The model under review builds one solid part; all positions refer to its coordinate system, in mm. A direction names the side the tool comes from. Round coordinates to 2 decimals unless told otherwise and drop trailing zeros. Write each loop counter-clockwise with the first axis right and the second up, starting at its lowest first coordinate (ties: lowest second). Pieces come first, ordered by that corner, then holes. Notation, with made-up numbers: (85.25, 50) -> (128.25, 50) arc R21 ccw to (128.25, 67) -> close; hole circle Ø8 at (55, 41.25). An arc over 180 degrees is marked (long way). Return JSON: item names as keys, results as strings. Group by question number.
1. Take a section at D-D, the plane x = 9. Write out the cut boundary in (y, z).
2. Take a section at A-A, the plane y = -4. Write out the cut boundary in (x, z).
3. Tool access review of faces 3 (the cylindrical face through (0.07, -3.53, 25.5)), 4 (the flat face through (35, 28.6, -20)): name each direction out of +Z, -Z, +X, -X, +Y, -Y from which nothing blocks a thin tool from reaching the whole face with its end or side.
4. For line 1 along Z through (x, y) = (4, -8); line 2 along Y through (x, z) = (-19, -38.5); line 3 along Y through (x, z) = (-32.5, 27), list the stretches that pass through material, from the lowest coordinate up. Write a range as from..to.
5. Take a section at C-C, the plane z = 41. Write out the cut boundary in (x, y), then the cut area to 3 significant figures.
6. Mouldability with a two-part tool opening along Z and no side actions: class faces 1 (the flat face through (-38.1, 22.1, 24.2)), 2 (the cylindrical face through (-4.88, -10.07, -1.08)) as pulls with the +Z half, pulls with the -Z half, needs draft (parallel to the pull), parting line crosses it, or undercut.
7. Clearance check with flat-ended pins moving along their axes: P1, Ø3.5, axis at x = 41.5, z = -0.5, coming from the +Y side; P2, Ø0.9, axis at x = -0.5, z = 27, coming from the +Y side; P3, Ø0.9, axis at x = -34, z = -20.5, coming from the +Y side. State where each tip first meets the part, or that it passes through.
8. Take a section at B-B, the plane y = -11. Write out the cut boundary in (x, z) (1 decimal), then the cut area to 3 significant figures.
from build123d import *

# Parameters (mm, degrees)
SHPERE_HULL_ANGLE    = 180
SKETCH3_W            = 50
SKETCH3_H            = 70
BATTERY_CAVITY_DEPTH = 18.3
SKETCH7_R            = 1.5
CUT_EXTRUDE4_DEPTH   = 12
PCB_START            = 6.5
SKETCH9_R            = 3.1
SKETCH9_R_2          = 1.5
PCB_STAND_OFFS_DEPTH = 6.5
SKETCH10_W           = 10
SKETCH10_H           = 3
BATTERY_CABLE_DEPTH  = 18.3
SKETCH20_R           = 44.9
SKETCH20_R_2         = 44.1
RAISED_LIP_DEPTH     = 1.6
SKETCH22_R           = 20
BALLAST_AREA_DEPTH   = 22
FILLET2_R            = 0.5
SKETCH23_R           = 1.5
THREADED_HOLES_DEPTH = 10
CIRPATTERN1_COUNT    = 4
SKETCH24_R           = 24
CUT_EXTRUDE5_DEPTH   = 2.4
SKETCH25_R           = 1.5
CUT_EXTRUDE6_DEPTH   = 10
SKETCH26_R           = 5
BOSS_EXTRUDE5_DEPTH  = 18.5
FILLET3_R            = 2


with BuildPart() as part:
    # Sketch19 → Shpere Hull (revolve)
    with BuildSketch(Plane(origin=(0, 22.1, 0), x_dir=(1, 0, 0), z_dir=(0, 1, 0))):
        with BuildLine():
            Line((0, 47), (0, -47))
            ThreePointArc((0, -47), (-47, 0), (0, 47))
        make_face()
    revolve(axis=Axis((0, 22.1, -47), (0, 0, 1)), revolution_arc=SHPERE_HULL_ANGLE)

    # Sketch3 → Battery Cavity (cut)
    with BuildSketch(Plane(origin=(0, 22.1, 0), x_dir=(1, 0, 0), z_dir=(0, 1, 0))):
        Rectangle(SKETCH3_W, SKETCH3_H)
    extrude(amount=-BATTERY_CAVITY_DEPTH, mode=Mode.SUBTRACT)

    # Sketch7 → Cut-Extrude4 (cut)
    with BuildSketch(Plane(origin=(0, 22.1, 0), x_dir=(1, 0, 0), z_dir=(0, 1, 0))):
        with Locations(Location((-33.25, 20.75, 0), (0, 0, 270))):
            Circle(SKETCH7_R)
        with Locations(Location((-33.25, -20.75, 0), (0, 0, 270))):
            Circle(SKETCH7_R)
        with Locations(Location((33.25, 20.75, 0), (0, 0, 270))):
            Circle(SKETCH7_R)
        with Locations(Location((33.25, -20.75, 0), (0, 0, 270))):
            Circle(SKETCH7_R)
    extrude(amount=-CUT_EXTRUDE4_DEPTH, mode=Mode.SUBTRACT)

    # Sketch9 → PCB Stand Offs (add)
    # profile 1 of 4: a face of its own
    with BuildSketch(Plane(origin=(0, 22.1, 0), x_dir=(1, 0, 0), z_dir=(0, 1, 0)).offset(PCB_START)):
        with Locations(Location((-33.25, 20.75, 0), (0, 0, 90))):
            Circle(SKETCH9_R)
        with Locations(Location((-33.25, 20.75, 0), (0, 0, 270))):
            Circle(SKETCH9_R_2, mode=Mode.SUBTRACT)
    # profile 2 of 4: a face of its own
    with BuildSketch(Plane(origin=(0, 22.1, 0), x_dir=(1, 0, 0), z_dir=(0, 1, 0)).offset(PCB_START)):
        with Locations(Location((33.25, 20.75, 0), (0, 0, 90))):
            Circle(SKETCH9_R)
        with Locations(Location((33.25, 20.75, 0), (0, 0, 270))):
            Circle(SKETCH9_R_2, mode=Mode.SUBTRACT)
    # profile 3 of 4: a face of its own
    with BuildSketch(Plane(origin=(0, 22.1, 0), x_dir=(1, 0, 0), z_dir=(0, 1, 0)).offset(PCB_START)):
        with Locations(Location((33.25, -20.75, 0), (0, 0, 90))):
            Circle(SKETCH9_R)
        with Locations(Location((33.25, -20.75, 0), (0, 0, 270))):
            Circle(SKETCH9_R_2, mode=Mode.SUBTRACT)
    # profile 4 of 4: a face of its own
    with BuildSketch(Plane(origin=(0, 22.1, 0), x_dir=(1, 0, 0), z_dir=(0, 1, 0)).offset(PCB_START)):
        with Locations(Location((-33.25, -20.75, 0), (0, 0, 90))):
            Circle(SKETCH9_R)
        with Locations(Location((-33.25, -20.75, 0), (0, 0, 270))):
            Circle(SKETCH9_R_2, mode=Mode.SUBTRACT)
    extrude(amount=-PCB_STAND_OFFS_DEPTH)

    # Sketch10 → Battery Cable (cut)
    with BuildSketch(Plane(origin=(0, 22.1, 0), x_dir=(1, 0, 0), z_dir=(0, 1, 0))):
        with Locations((-14, 36.5)):
            Rectangle(SKETCH10_W, SKETCH10_H)
    extrude(amount=-BATTERY_CABLE_DEPTH, mode=Mode.SUBTRACT)

    # Sketch20 → Raised Lip (add)
    with BuildSketch(Plane(origin=(0, 22.1, 0), x_dir=(1, 0, 0), z_dir=(0, 1, 0))):
        Circle(SKETCH20_R)
        with Locations(Location((0, 0, 0), (0, 0, 180))):
            Circle(SKETCH20_R_2, mode=Mode.SUBTRACT)
    extrude(amount=RAISED_LIP_DEPTH)

    # Sketch22 → Ballast Area (cut)
    with BuildSketch(Plane(origin=(0, 3.8, 0), x_dir=(1, 0, 0), z_dir=(0, 1, 0))):
        with Locations(Location((0, 0, 0), (0, 0, 270))):
            Circle(SKETCH22_R)
    extrude(amount=-BALLAST_AREA_DEPTH, mode=Mode.SUBTRACT)

    # Fillet2
    fillet2_edges = [part.edges().sort_by_distance(p)[0] for p in [
        (-25, 12.95, 35),
        (-25, 12.95, -35),
        (25, 12.95, -35),
        (25, 12.95, 35),
        (-19, 12.95, -35),
        (-19, 12.95, -38),
        (-9, 12.95, -38),
        (-9, 12.95, -35),
    ]]
    fillet(fillet2_edges, radius=FILLET2_R)

    # Sketch23 → Threaded Holes (cut)
    with BuildSketch(Plane(origin=(0, 22.1, 0), x_dir=(1, 0, 0), z_dir=(0, 1, 0))):
        with Locations(Location((0, 41, 0), (0, 0, 180))):
            Circle(SKETCH23_R)
        with Locations(Location((0, -41, 0), (0, 0, 180))):
            Circle(SKETCH23_R)
    threaded_holes = extrude(amount=-THREADED_HOLES_DEPTH, mode=Mode.SUBTRACT)

    # CirPattern1: Threaded Holes ×4 about axis
    cirpattern1_axis = Axis((0, 0, 0), (0, 1, 0))
    for i in range(1, CIRPATTERN1_COUNT):
        add(threaded_holes.rotate(cirpattern1_axis, i * 360 / CIRPATTERN1_COUNT), mode=Mode.SUBTRACT)

    # Sketch24 → Cut-Extrude5 (cut)
    with BuildSketch(Plane(origin=(0, 3.8, 0), x_dir=(1, 0, 0), z_dir=(0, 1, 0))):
        Circle(SKETCH24_R)
        with BuildLine():
            Line((3, -31), (-3, -31))
            ThreePointArc((-3, -31), (-5.121320344, -30.121320344), (-6, -28))
            Line((-6, -28), (-6, 28))
            ThreePointArc((-6, 28), (-5.121320344, 30.121320344), (-3, 31))
            Line((-3, 31), (3, 31))
            ThreePointArc((3, 31), (5.121320344, 30.121320344), (6, 28))
            Line((6, 28), (6, -28))
            ThreePointArc((6, -28), (5.121320344, -30.121320344), (3, -31))
        make_face()
    extrude(amount=-CUT_EXTRUDE5_DEPTH, mode=Mode.SUBTRACT)

    # Sketch25 → Cut-Extrude6 (cut)
    with BuildSketch(Plane(origin=(0, 1.4, 0), x_dir=(1, 0, 0), z_dir=(0, 1, 0))):
        with Locations(Location((0, 27, 0), (0, 0, 270))):
            Circle(SKETCH25_R)
        with Locations(Location((0, -27, 0), (0, 0, 270))):
            Circle(SKETCH25_R)
    extrude(amount=-CUT_EXTRUDE6_DEPTH, mode=Mode.SUBTRACT)

    # Sketch26 → Boss-Extrude5 (add)
    with BuildSketch(Plane(origin=(0, -18.2, 0), x_dir=(1, 0, 0), z_dir=(0, 1, 0))):
        with Locations(Location((0, 0, 0), (0, 0, 270))):
            Circle(SKETCH26_R)
    extrude(amount=BOSS_EXTRUDE5_DEPTH)

    # Fillet3
    fillet3_edges = [part.edges().sort_by_distance(p)[0] for p in [
        (0, 0.3, -5),
    ]]
    fillet(fillet3_edges, radius=FILLET3_R)


solid = part.part
Output:
{
 "1": {"outline": "(-18.2, -17.86) -> (-18.2, 17.86) -> (1.4, 17.86) -> (1.4, 22.25) -> (3.8, 22.25) -> (3.8, 35) -> (22.1, 35) -> (22.1, 43.17) -> (23.7, 43.17) -> (23.7, 43.99) -> (22.1, 43.99) -> (22.1, 46.13) arc R46.13 ccw to (22.1, -46.13) -> (22.1, -43.99) -> (23.7, -43.99) -> (23.7, -43.17) -> (22.1, -43.17) -> (22.1, -35) -> (3.8, -35) -> (3.8, -22.25) -> (1.4, -22.25) -> (1.4, -17.86) -> close"},
 "2": {"outline": "circle Ø78.17 at (0, 0); circle Ø10 at (0, 0); hole circle Ø40 at (0, 0); hole circle Ø3 at (0, -27); hole circle Ø3 at (0, 27)"},
 "3": {"face 3": "+Y", "face 4": "+Z, -Z, +X, -X, +Y"},
 "4": {"line 1": "z = -35.87..-19.6, -3..3, 19.6..35.87", "line 2": "y = 2.98..22.1", "line 3": "y = 1.51..22.1"},
 "5": {"outline": "(-22.98, 22.1) arc R22.98 ccw to (22.98, 22.1) -> (18.3, 22.1) -> (18.3, 23.7) -> (16.24, 23.7) -> (16.24, 22.1) -> (1.5, 22.1) -> (1.5, 12.1) -> (-1.5, 12.1) -> (-1.5, 22.1) -> (-16.24, 22.1) -> (-16.24, 23.7) -> (-18.3, 23.7) -> (-18.3, 22.1) -> close", "area": "806 mm^2"},
 "6": {"face 1": "needs draft", "face 2": "undercut"},
 "7": {"P1": "stops at y = 22.1", "P2": "stops at y = -8.6", "P3": "stops at y = 10.1"},
 "8": {"outline": "circle Ø66.7 at (0, 0); circle Ø10 at (0, 0); hole circle Ø40 at (0, 0)", "area": "2,320 mm^2"}
}
